Check sheet for the modelled part. Datum: model origin and axes. Units: mm. Coordinates: 2 decimals unless noted, no trailing zeros. Write each loop counter-clockwise with the first axis right and the second up, starting at its lowest first coordinate (ties: lowest second). Pieces come first, ordered by that corner, then holes. Notation, with made-up numbers: (-20, 56) -> (-9, 56) arc R16 cw to (-9, 72) -> close; hole circle Ø7 at (63.5, 54). An arc over 180 degrees is marked (long way). Put each result on its own line as item: value.
```python
from build123d import *

# Parameters (mm, degrees)
SKETCH_1_R          = 5.05
SKETCH_1_R_2        = 13
EXTRUDE_1_DEPTH     = 15
FILLET_1_R          = 3
CUT_EXTRUDE_3_DEPTH = 277.54113618
FILLET_2_R          = 3
EXTRUDE_3_DEPTH     = 15
FILLET_4_R          = 3
SKETCH_8_R          = 13
CUT_EXTRUDE_5_DEPTH = 277.54113618
SKETCH_9_R          = 25
SKETCH_9_R_2        = 13
EXTRUDE_4_DEPTH     = 15


with BuildPart() as part:
    # 草图1 → 凸台-拉伸1 (new body)
    with BuildSketch(Plane(origin=(0, 0, 0), x_dir=(1, 0, 0), z_dir=(0, 1, 0))):
        with BuildLine():
            Line((-17.992942616, -0.504), (-24.990198078, 249.3))
            ThreePointArc((-24.990198078, 249.3), (0, 275), (24.990198078, 249.3))
            Line((24.990198078, 249.3), (17.992942616, -0.504))
            ThreePointArc((17.992942616, -0.504), (0, -18), (-17.992942616, -0.504))
        make_face()
        with Locations(Location((0, 0, 0), (0, 0, 270))):
            Circle(SKETCH_1_R, mode=Mode.SUBTRACT)
        with Locations(Location((0, 250, 0), (0, 0, 270))):
            Circle(SKETCH_1_R_2, mode=Mode.SUBTRACT)
        Polygon((-16.444447487, 158.5), (-17.704941698, 203.5), (11.028871219, 137.174942267), align=None, mode=Mode.SUBTRACT)
        Polygon((15.954255294, 141), (18.475243716, 231), (-12, 219.5), align=None, mode=Mode.SUBTRACT)
    extrude(amount=EXTRUDE_1_DEPTH)

    # 圆角1
    fillet_1_edges = [part.edges().sort_by_distance(p)[0] for p in [
        (-16.444447487, 7.5, -158.5),
        (11.028871219, 7.5, -137.174942267),
        (-17.704941698, 7.5, -203.5),
        (18.475243716, 7.5, -231),
        (-12, 7.5, -219.5),
        (15.954255294, 7.5, -141),
    ]]
    fillet(fillet_1_edges, radius=FILLET_1_R)

    # 草图4 → 切除-拉伸3 (cut, through all)
    with BuildSketch(Plane(origin=(0, 15, 0), x_dir=(1, 0, 0), z_dir=(0, 1, 0))):
        Polygon((-13.050343026, 144.472367448), (12.494927596, 124.643879429), (9.742058902, 26.365688077), (-10.175105816, 41.825585442), align=None)
    extrude(amount=-CUT_EXTRUDE_3_DEPTH, mode=Mode.SUBTRACT)

    # 圆角2
    fillet_2_edges = [part.edges().sort_by_distance(p)[0] for p in [
        (-10.175105816, 7.5, -41.825585442),
        (-13.050343026, 7.5, -144.472367448),
        (9.742058902, 7.5, -26.365688077),
    ]]
    fillet(fillet_2_edges, radius=FILLET_2_R)

    # 草图6 → 凸台-拉伸3 (add)
    with BuildSketch(Plane(origin=(0, 15, 0), x_dir=(1, 0, 0), z_dir=(0, 1, 0))):
        Polygon((9.60137553, 125.435937788), (-13.068657882, 42.617643801), (-7.609801347, 39.834371112), (-7.28155375, 41.033527083), (15.388479662, 123.85182107), (9.929623127, 126.635093759), align=None)
    extrude(amount=-EXTRUDE_3_DEPTH)

    # 圆角4
    fillet_4_edges = [part.edges().sort_by_distance(p)[0] for p in [
        (9.929623127, 7.5, -126.635093759),
        (12.14036175, 7.5, -111.985778385),
        (-7.609801347, 7.5, -39.834371112),
        (-10.463842583, 7.5, -52.133569747),
    ]]
    fillet(fillet_4_edges, radius=FILLET_4_R)

    # 草图8 → 切除-拉伸5 (cut, through all)
    with BuildSketch(Plane(origin=(0, 15, 0), x_dir=(1, 0, 0), z_dir=(0, 1, 0))):
        with Locations(Location((0, 0, 0), (0, 0, 270))):
            Circle(SKETCH_8_R)
    extrude(amount=-CUT_EXTRUDE_5_DEPTH, mode=Mode.SUBTRACT)

    # 草图9 → 凸台-拉伸4 (add)
    with BuildSketch(Plane(origin=(0, 15, 0), x_dir=(1, 0, 0), z_dir=(0, 1, 0))):
        Circle(SKETCH_9_R)
        with Locations(Location((0, 0, 0), (0, 0, 270))):
            Circle(SKETCH_9_R_2, mode=Mode.SUBTRACT)
    extrude(amount=-EXTRUDE_4_DEPTH)


solid = part.part
```
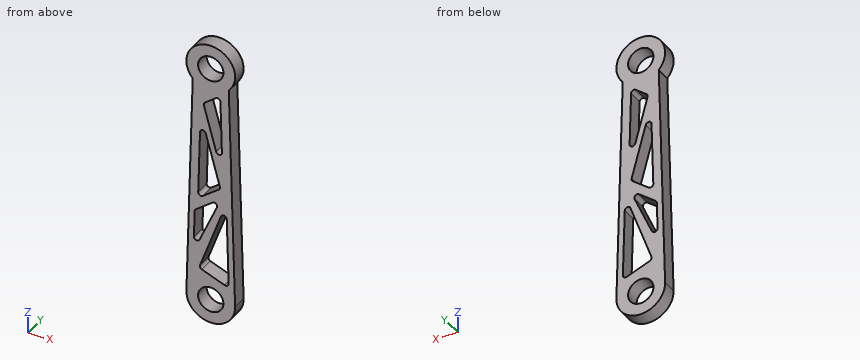
Q1. Cross-section at A-A (z = 0). Record the cut outline in (x, y).
Recorded:
outline: (-25, 0) -> (-13, 0) -> (-13, 15) -> (-25, 15) -> close; (13, 0) -> (25, 0) -> (25, 15) -> (13, 15) -> close
Q2. Cross-section at D-D (z = -107). Record the cut outline in (x, y).
Recorded:
outline: (-21, 0) -> (-12, 0) -> (-12, 15) -> (-21, 15) -> close; (4.55, 0) -> (21, 0) -> (21, 15) -> (4.55, 15) -> close
Q3. Material ranges on line 1 along X through (y, z) = (9.5, 0); line 2 along X through (y, z) = (8, -77); line 3 along X through (y, z) = (13.75, -261), recorded low to high.
Recorded:
line 1: x = -25 to -13, 13 to 25
line 2: x = -20.16 to -11.16, -3.66 to 2.56, 11.16 to 20.16
line 3: x = -22.45 to -6.93, 6.93 to 22.45
Q4. Cross-section at B-B (z = -75). Record the cut outline in (x, y), plus the area to 3 significant figures.
Recorded:
outline: (-20.11, 0) -> (-11.1, 0) -> (-11.1, 15) -> (-20.11, 15) -> close; (-4.2, 0) -> (2.02, 0) -> (2.02, 15) -> (-4.2, 15) -> close; (11.1, 0) -> (20.11, 0) -> (20.11, 15) -> (11.1, 15) -> close
area: 363 mm2
Q5. Cross-section at C-C (y = 11.75). State how many separate pieces and enclosed holes the cut face has, plus the area to 3 significant figures.
Recorded:
separate pieces: 1
enclosed holes: 6
area: 8,280 mm2
Q6. Depth check by flat-ended pin: P1, Ø4, axis at y = 11, z = -176, coming from the +X side; P2, Ø3, axis at y = 4, z = -105.5, coming from the -X side; P3, Ø8, axis at y = 6.5, z = -111, coming from the -X side. Enter the tip coordinate at first touch or a pass-through.
Recorded:
P1: stops at x = 22.99
P2: stops at x = -21
P3: stops at x = -21.23
